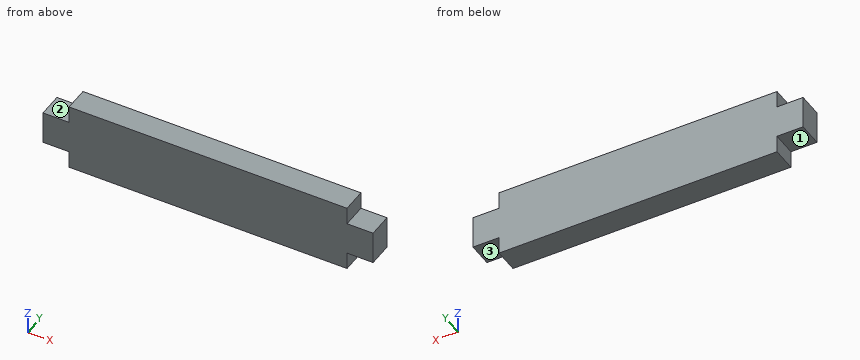
from build123d import *

# Parameters (mm, degrees)
SKETCH2_W           = 80
SKETCH2_H           = 7
BOSS_EXTRUDE1_DEPTH = 19.5
SKETCH3_W           = 7.5
SKETCH3_H           = 9.5
BOSS_EXTRUDE2_DEPTH = 7


with BuildPart() as part:
    # Sketch2 → Boss-Extrude1 (new body)
    with BuildSketch(Plane.XY):
        with Locations((40, -3.5)):
            Rectangle(SKETCH2_W, SKETCH2_H)
    extrude(amount=BOSS_EXTRUDE1_DEPTH)

    # Sketch3 → Boss-Extrude2 (add)
    with BuildSketch(Plane(origin=(0, 0, 0), x_dir=(1, 0, 0), z_dir=(0, 1, 0))):
        with Locations((-3.75, -9.75)):
            Rectangle(SKETCH3_W, SKETCH3_H)
        with Locations((83.75, -9.75)):
            Rectangle(SKETCH3_W, SKETCH3_H)
    extrude(amount=-BOSS_EXTRUDE2_DEPTH)


solid = part.part
Read the model definition and answer for the solid it produces. Units are mm, in the model's axes. Face numbers are marked on the shaded views. A direction names the side the tool comes from. Round coordinates to 2 decimals unless told otherwise and drop trailing zeros. Write each loop counter-clockwise with the first axis right and the second up, starting at its lowest first coordinate (ties: lowest second). Pieces come first, ordered by that corner, then holes. Notation, with made-up numbers: (13, -28.5) - (31, -28.5) arc R25 ccw to (31, -11.5) - close; hole circle Ø2 at (56.25, 89). An arc over 180 degrees is marked (long way). Use a Markdown table: item, result.
(1) Each of these flat-tipped pins is pushed along its axis until it touches: pin 1 Ø2.5 at (y, z) = (-3.5, 16.5) entering from -X; pin 2 Ø2.5 at (y, z) = (-5, 3) entering from +X; pin 3 Ø3.5 at (x, y) = (82.5, -4) entering from +Z. Where does it stop, or does it pass through?
Reported:
| item | result |
|---|---|
| pin 1 | x = 0 |
| pin 2 | x = 80 |
| pin 3 | z = 14.5 |
(2) Straight lines are drawn through the part: line 1 along X through (y, z) = (-3.5, 18.5); line 2 along Z through (x, y) = (81.5, -6.25). For each, find the intervals that lie inside material, in ascending order. Write a range as [from, to].
Reported:
| item | result |
|---|---|
| line 1 | [0, 80] |
| line 2 | [5, 14.5] |
(3) The part is cut by section C-C (x = 82.5). Write down the section's boundary in (y, z), then the cut area to 3 significant figures.
Reported:
| item | result |
|---|---|
| outline | (-7, 5) - (0, 5) - (0, 14.5) - (-7, 14.5) - close |
| area | 66.5 mm2 |
(4) The part is cut by section B-B (z = 16). Write down the section's boundary in (x, y), then the cut area to 3 significant figures.
Reported:
| item | result |
|---|---|
| outline | (0, -7) - (80, -7) - (80, 0) - (0, 0) - close |
| area | 560 mm2 |
(5) Which of the six approach directions +Z, -Z, +X, -X, +Y, -Y give full straight-line access (tool end or side, diameter ignored) to the marked faces 1, 2 and 3?
Reported:
| item | result |
|---|---|
| face 1 | -Z, -X, +Y, -Y |
| face 2 | +Z, -X, +Y, -Y |
| face 3 | -Z, +X, +Y, -Y |
(6) The part is cut by section A-A (y = -2.5). Write down the section's boundary in (x, z), then the cut area to 3 significant figures.
Reported:
| item | result |
|---|---|
| outline | (-7.5, 5) - (0, 5) - (0, 0) - (80, 0) - (80, 5) - (87.5, 5) - (87.5, 14.5) - (80, 14.5) - (80, 19.5) - (0, 19.5) - (0, 14.5) - (-7.5, 14.5) - close |
| area | 1,700 mm2 |
